Source: CAD feature listing. Evaluate the final solid. Frame: model axes, mm. Face numbers are marked on the shaded views. A direction names the side the tool comes from. Give positions to 0.01 mm unless a question says otherwise; leave off trailing zeros. Loops run counter-clockwise (first coordinate to the right, second up) from the corner with the lowest first, then second, coordinate; pieces in that order, holes last.
from build123d import *

# Parameters (mm, degrees)
SKETCH1_W            = 112
SKETCH1_H            = 106
BOSS_EXTRUDE1_DEPTH  = 3
SKETCH3_W            = 112
SKETCH3_H            = 106
BOSS_EXTRUDE2_DEPTH  = 30
CUT_EXTRUDE1_DEPTH   = 15
SKETCH5_R            = 1
SKETCH5_W            = 16
SKETCH5_H            = 6
CUT_EXTRUDE2_DEPTH   = 3
SKETCH7_W            = 30
SKETCH7_H            = 14.5
CUT_EXTRUDE4_DEPTH   = 112
SKETCH9_W            = 112
SKETCH9_H            = 20
BOSS_EXTRUDE3_DEPTH  = 3
SKETCH10_W           = 11
SKETCH10_H           = 18
CUT_EXTRUDE5_DEPTH   = 13.5
BOSS_EXTRUDE4_DEPTH  = 112
BOSS_EXTRUDE5_DEPTH  = 3
BOSS_EXTRUDE6_DEPTH  = 3
SKETCH19_W           = 9
SKETCH19_H           = 10
CUT_EXTRUDE7_DEPTH   = 3
SKETCH20_W           = 12
SKETCH20_H           = 13
SKETCH20_W_2         = 9
SKETCH20_H_2         = 10
BOSS_EXTRUDE8_DEPTH  = 3
SKETCH21_W           = 15
SKETCH21_H           = 8.5
CUT_EXTRUDE8_DEPTH   = 3
SKETCH23_W           = 25
SKETCH23_H           = 1.5
CUT_EXTRUDE9_DEPTH   = 3
SKETCH24_W           = 25
SKETCH24_H           = 1.5
CUT_EXTRUDE10_DEPTH  = 3
FILLET1_R            = 1.5
SKETCH31_W           = 2
SKETCH31_H           = 10.5
BOSS_EXTRUDE16_DEPTH = 10


with BuildPart() as part:
    # Sketch1 → Boss-Extrude1 (new body)
    with BuildSketch(Plane(origin=(0, 0, 0), x_dir=(1, 0, 0), z_dir=(0, 1, 0))):
        Rectangle(SKETCH1_W, SKETCH1_H)
    extrude(amount=BOSS_EXTRUDE1_DEPTH)

    # Sketch3 → Boss-Extrude2 (add)
    with BuildSketch(Plane.XZ):
        Rectangle(SKETCH3_W, SKETCH3_H)
        with BuildLine():
            ThreePointArc((-44.381049961, -50), (-47.452820621, -44.577071492), (-52.830188679, -41.426223771))
            Line((-52.830188679, -41.426223771), (-52.830188679, 41.426223771))
            ThreePointArc((-52.830188679, 41.426223771), (-47.452820621, 44.577071492), (-44.381049961, 50))
            Line((-44.381049961, 50), (44.381049961, 50))
            ThreePointArc((44.381049961, 50), (47.452820621, 44.577071492), (52.830188679, 41.426223771))
            Line((52.830188679, 41.426223771), (52.830188679, -41.426223771))
            ThreePointArc((52.830188679, -41.426223771), (47.452820621, -44.577071492), (44.381049961, -50))
            Line((44.381049961, -50), (-44.381049961, -50))
        make_face(mode=Mode.SUBTRACT)
    extrude(amount=BOSS_EXTRUDE2_DEPTH)

    # Sketch4 → Cut-Extrude1 (cut)
    with BuildSketch(Plane.XZ.offset(30)):
        with BuildLine():
            ThreePointArc((-50, 48.5), (-52.560660172, 49.560660172), (-51.5, 47))
            Line((-51.5, 47), (-51.5, 48.5))
            Line((-51.5, 48.5), (-50, 48.5))
        make_face()
        with BuildLine():
            Line((-51.5, 48.5), (-51.5, 47))
            ThreePointArc((-51.5, 47), (-50.439339828, 47.439339828), (-50, 48.5))
            Line((-50, 48.5), (-51.5, 48.5))
        make_face()
        with BuildLine():
            Line((-51.5, -47), (-51.5, -48.5))
            Line((-51.5, -48.5), (-50, -48.5))
            ThreePointArc((-50, -48.5), (-50.439339828, -47.439339828), (-51.5, -47))
        make_face()
        with BuildLine():
            Line((-50, -48.5), (-51.5, -48.5))
            Line((-51.5, -48.5), (-51.5, -47))
            ThreePointArc((-51.5, -47), (-52.560660172, -49.560660172), (-50, -48.5))
        make_face()
        with BuildLine():
            ThreePointArc((51.5, -47), (50.439339828, -47.439339828), (50, -48.5))
            Line((50, -48.5), (51.5, -48.5))
            Line((51.5, -48.5), (51.5, -47))
        make_face()
        with BuildLine():
            Line((51.5, -48.5), (50, -48.5))
            ThreePointArc((50, -48.5), (51.5, -50), (53, -48.5))
            ThreePointArc((53, -48.5), (52.560660172, -47.439339828), (51.5, -47))
            Line((51.5, -47), (51.5, -48.5))
        make_face()
        with BuildLine():
            ThreePointArc((50, 48.5), (50.439339828, 47.439339828), (51.5, 47))
            Line((51.5, 47), (51.5, 48.5))
            Line((51.5, 48.5), (50, 48.5))
        make_face()
        with BuildLine():
            Line((51.5, 48.5), (51.5, 47))
            ThreePointArc((51.5, 47), (52.560660172, 47.439339828), (53, 48.5))
            ThreePointArc((53, 48.5), (51.5, 50), (50, 48.5))
            Line((50, 48.5), (51.5, 48.5))
        make_face()
    extrude(amount=-CUT_EXTRUDE1_DEPTH, mode=Mode.SUBTRACT)

    # Sketch5 → Cut-Extrude2 (cut)
    with BuildSketch(Plane.XY.offset(53)):
        with Locations((9.5, -19)):
            Circle(SKETCH5_R)
        with Locations((-9.5, -19)):
            Circle(SKETCH5_R)
        with Locations((0, -19)):
            Rectangle(SKETCH5_W, SKETCH5_H)
    extrude(amount=-CUT_EXTRUDE2_DEPTH, mode=Mode.SUBTRACT)

    # Sketch7 → Cut-Extrude4 (cut)
    with BuildSketch(Plane(origin=(56, 0, 0), x_dir=(0, 0, -1), z_dir=(1, 0, 0))):
        with Locations((-38, -4.25)):
            Rectangle(SKETCH7_W, SKETCH7_H)
    extrude(amount=-CUT_EXTRUDE4_DEPTH, mode=Mode.SUBTRACT)

    # Sketch9 → Boss-Extrude3 (add)
    with BuildSketch(Plane(origin=(0, -11.5, 0), x_dir=(1, 0, 0), z_dir=(0, 1, 0))):
        with Locations((0, -43)):
            Rectangle(SKETCH9_W, SKETCH9_H)
    extrude(amount=BOSS_EXTRUDE3_DEPTH)

    # Sketch10 → Cut-Extrude5 (cut)
    with BuildSketch(Plane(origin=(0, -8.5, 0), x_dir=(1, 0, 0), z_dir=(0, 1, 0))):
        with Locations((-22, -44)):
            Rectangle(SKETCH10_W, SKETCH10_H)
        with Locations((22, -44)):
            Rectangle(SKETCH10_W, SKETCH10_H)
    extrude(amount=-CUT_EXTRUDE5_DEPTH, mode=Mode.SUBTRACT)

    # Sketch11 → Boss-Extrude4 (add)
    with BuildSketch(Plane(origin=(56, 0, 0), x_dir=(0, 0, -1), z_dir=(1, 0, 0))):
        Polygon((-33, -8.5), (-23, 3), (-23, 0), (-33, -11.5), align=None)
    extrude(amount=-BOSS_EXTRUDE4_DEPTH)

    # Sketch13 → Boss-Extrude5 (add)
    with BuildSketch(Plane(origin=(56, 0, 0), x_dir=(0, 0, -1), z_dir=(1, 0, 0))):
        Polygon((-33, -11.5), (-23, 0), (-23, -11.5), align=None)
    extrude(amount=-BOSS_EXTRUDE5_DEPTH)

    # Sketch14 → Boss-Extrude6 (add)
    with BuildSketch(Plane.ZY.offset(56)):
        Polygon((23, 0), (23, -11.5), (33, -11.5), align=None)
    extrude(amount=-BOSS_EXTRUDE6_DEPTH)

    # Sketch19 → Cut-Extrude7 (cut)
    with BuildSketch(Plane(origin=(0, 0, -53), x_dir=(-1, 0, 0), z_dir=(0, 0, -1))):
        with Locations((23, -16.5)):
            Rectangle(SKETCH19_W, SKETCH19_H)
    extrude(amount=-CUT_EXTRUDE7_DEPTH, mode=Mode.SUBTRACT)

    # Sketch20 → Boss-Extrude8 (add)
    with BuildSketch(Plane.XY.offset(-53)):
        with Locations((-23, -16.5)):
            Rectangle(SKETCH20_W, SKETCH20_H)
        with Locations((-23, -16.5)):
            Rectangle(SKETCH20_W_2, SKETCH20_H_2, mode=Mode.SUBTRACT)
    extrude(amount=BOSS_EXTRUDE8_DEPTH)

    # Sketch21 → Cut-Extrude8 (cut)
    with BuildSketch(Plane(origin=(0, 0, -53), x_dir=(-1, 0, 0), z_dir=(0, 0, -1))):
        with Locations((-21, -15)):
            Rectangle(SKETCH21_W, SKETCH21_H)
    extrude(amount=-CUT_EXTRUDE8_DEPTH, mode=Mode.SUBTRACT)

    # Sketch23 → Cut-Extrude9 (cut)
    with BuildSketch(Plane(origin=(56, 0, 0), x_dir=(0, 0, -1), z_dir=(1, 0, 0))):
        with Locations((32.5, -8.75)):
            Rectangle(SKETCH23_W, SKETCH23_H)
        with Locations((32.5, -3.75)):
            Rectangle(SKETCH23_W, SKETCH23_H)
        with Locations((32.5, -13.75)):
            Rectangle(SKETCH23_W, SKETCH23_H)
        with Locations((32.5, -18.75)):
            Rectangle(SKETCH23_W, SKETCH23_H)
        with Locations((32.5, -23.75)):
            Rectangle(SKETCH23_W, SKETCH23_H)
        with Locations((-2.5, -23.75)):
            Rectangle(SKETCH23_W, SKETCH23_H)
        with Locations((-2.5, -18.75)):
            Rectangle(SKETCH23_W, SKETCH23_H)
        with Locations((-2.5, -13.75)):
            Rectangle(SKETCH23_W, SKETCH23_H)
        with Locations((-2.5, -8.75)):
            Rectangle(SKETCH23_W, SKETCH23_H)
        with Locations((-2.5, -3.75)):
            Rectangle(SKETCH23_W, SKETCH23_H)
    extrude(amount=-CUT_EXTRUDE9_DEPTH, mode=Mode.SUBTRACT)

    # Sketch24 → Cut-Extrude10 (cut)
    with BuildSketch(Plane.ZY.offset(56)):
        with Locations((2.5, -7.25)):
            Rectangle(SKETCH24_W, SKETCH24_H)
        with Locations((2.5, -3.75)):
            Rectangle(SKETCH24_W, SKETCH24_H)
        with Locations((2.5, -12.25)):
            Rectangle(SKETCH24_W, SKETCH24_H)
        with Locations((2.5, -17.25)):
            Rectangle(SKETCH24_W, SKETCH24_H)
        with Locations((2.5, -22.25)):
            Rectangle(SKETCH24_W, SKETCH24_H)
        with Locations((-32.5, -22.25)):
            Rectangle(SKETCH24_W, SKETCH24_H)
        with Locations((-32.5, -17.25)):
            Rectangle(SKETCH24_W, SKETCH24_H)
        with Locations((-32.5, -12.25)):
            Rectangle(SKETCH24_W, SKETCH24_H)
        with Locations((-32.5, -7.25)):
            Rectangle(SKETCH24_W, SKETCH24_H)
        with Locations((-32.5, -3.75)):
            Rectangle(SKETCH24_W, SKETCH24_H)
    extrude(amount=-CUT_EXTRUDE10_DEPTH, mode=Mode.SUBTRACT)

    # Fillet1
    fillet1_edges = [part.edges().sort_by_distance(p)[0] for p in [
        (56, 3, -15),
        (-56, -19.25, 53),
        (56, -19.25, 53),
        (0, 3, 23),
        (-56, 3, -15),
        (-56, -8.5, 43),
        (-41.75, -8.5, 53),
        (56, -8.5, 43),
        (0, -8.5, 33),
        (0, -8.5, 53),
        (41.75, -8.5, 53),
        (-56, -2.75, 28),
        (56, -2.75, 28),
        (-56, -13.5, -53),
        (56, -13.5, -53),
        (0, 3, -53),
    ]]
    fillet(fillet1_edges, radius=FILLET1_R)

    # Sketch31 → Boss-Extrude16 (add)
    with BuildSketch(Plane(origin=(0, 0, 50), x_dir=(-1, 0, 0), z_dir=(0, 0, -1))):
        with Locations((-28.5, -16.75)):
            Rectangle(SKETCH31_W, SKETCH31_H)
        Polygon((-27.5, -22), (-29.5, -22), (-29.5, -23.5), (-14.5, -23.5), (-14.5, -22), (-16.5, -22), align=None)
        with Locations((-15.5, -16.75)):
            Rectangle(SKETCH31_W, SKETCH31_H)
        Polygon((16.5, -11.5), (14.5, -11.5), (14.5, -22), (14.5, -23.5), (29.5, -23.5), (29.5, -22), (29.5, -11.5), (27.5, -11.5), (27.5, -22), (16.5, -22), align=None)
    extrude(amount=BOSS_EXTRUDE16_DEPTH)


solid = part.part
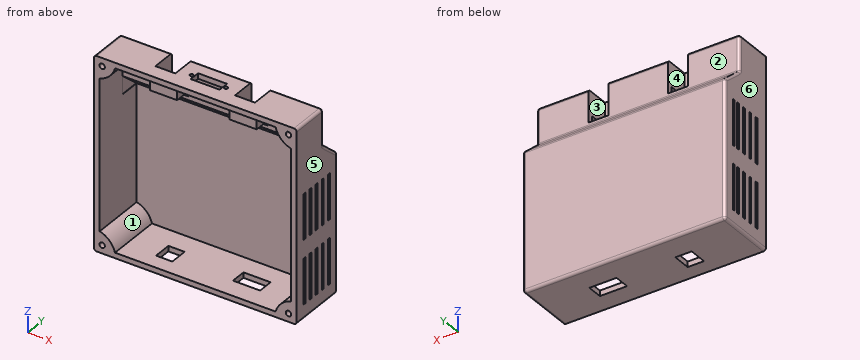
1) Contact query for flat-ended pins moving along their axis: P1, Ø1.2, axis at x = 54, y = -3.5, coming from the +Z side; P2, Ø5, axis at y = -7, z = 30.5, coming from the -X side; P3, Ø6, axis at x = -14.5, z = -9, coming from the -Y side. Output: stop coordinate, or through.
Checks:
P1: stops at z = 29.17
P2: stops at x = -56
P3: stops at y = 0
2) Cut plane B-B (x = -35). Return loops of the section in (y, z).
Checks:
outline: (-30, -53) - (1.5, -53) arc R1.5 ccw to (3, -51.5) - (3, 22.32) arc R1.5 ccw to (2.48, 23.45) - (-7.98, 32.55) arc R1.5 cw to (-8.5, 33.68) - (-8.5, 51.5) arc R1.5 ccw to (-10, 53) - (-30, 53) - (-30, 50) - (-11.5, 50) - (-11.5, 33) - (0, 23) - (0, -50) - (-30, -50) - close
3) Cut plane A-A (x = 25.5). Return loops of the section in (y, z).
Checks:
outline: (-30, -53) - (-19.25, -53) - (-19.25, -50) - (-30, -50) - close; (-30, 50) - (-23.5, 50) - (-23.5, 40) - (-22, 40) - (-22, 53) - (-30, 53) - close; (-11.5, 33) - (0, 23) - (0, -50) - (-10.75, -50) - (-10.75, -53) - (1.5, -53) arc R1.5 ccw to (3, -51.5) - (3, 22.32) arc R1.5 ccw to (2.48, 23.45) - (-7.98, 32.55) arc R1.5 cw to (-8.5, 33.68) - (-8.5, 35) - (-11.5, 35) - close
4) Pull-direction query (X, two-part tool) for the marked faces 4, 5 and 6; classes: released by +X, released by -X, zero draft, split by the parting line, or undercut.
Checks:
face 4: undercut
face 5: released by +X
face 6: released by -X
5) Reachability of the marked faces 1, 2 and 3 from +Z, -Z, +X, -X, +Y, -Y: full face, straight path, thin tool, end or side. Return the list, or none.
Checks:
face 1: -Y
face 2: +Z, +X, -X, +Y
face 3: +Z, +Y
6) Ray query, probe 1 along Z at (x, y) = (-14, -19); probe 2 along X at (y, z) = (-9, 14.5); probe 3 along X at (y, z) = (-6, 25). Return the intervals inside material, ascending.
Checks:
probe 1: z = -53 to -50, 50 to 53
probe 2: x = -56 to -52.83, 52.83 to 53
probe 3: x = -56 to -53, 53 to 56
